Autodesk Inventor part; units mm, degrees
ref_plane "YZ Plane" through (0, 0, 0) normal (1, 0, 0) x (0, 1, 0)
ref_plane "XZ Plane" through (0, 0, 0) normal (0, 1, 0) x (-1, 0, 0)
ref_plane "XY Plane" through (0, 0, 0) normal (0, 0, 1) x (1, 0, 0)
sketch "Sketch1" plane through (0, 0, 0) normal (0, 0, 1) x (1, 0, 0)
  circle A0 centre (0, 0) radius 12
  circle A1 centre (0, 0) radius 9 construction
  circle A2 centre (9, 0) radius 1.5
  circle A3 centre (-4.5, -7.7942) radius 1.5
  circle A4 centre (-4.5, 7.7942) radius 1.5
  line L0 (9, 0) -> (-4.5, -7.7942) construction
  line L1 (-4.5, 7.7942) -> (-4.5, -7.7942) construction
  line L2 (9, 0) -> (-4.5, 7.7942) construction
  circle A5 centre (0, 0) radius 2.5
  dimension "d0" = 24
  dimension "d1" = 18
  dimension "d2" = 3
  dimension "d3" = 5
extrude "Extrusion1" add sketch "Sketch1" along normal blind 5
sketch "Sketch2" plane through (0, 0, 5) normal (0, 0, 1) x (1, 0, 0)
  circle A0 centre (9, 0) radius 2.5
  circle A1 centre (-4.5, 7.7942) radius 2.5
  circle A2 centre (-4.5, -7.7942) radius 2.5
  circle A3 centre (9, 0) radius 1.5
  circle A4 centre (-4.5, -7.7942) radius 1.5
  circle A5 centre (-4.5, 7.7942) radius 1.5
  circle A6 centre (0, 0) radius 4
  circle A7 centre (0, 0) radius 2.5
  circle A8 centre (0, 0) radius 6.5
  dimension "d6" = 5
  dimension "d7" = 8
  dimension "d12" = 13
extrude "Extrusion2" cut sketch "Sketch2" against normal blind 3 contours A0 | A2 | A1 | A5
extrude "Extrusion3" add sketch "Sketch2" along normal blind 9 contours A6
sketch "Sketch3" plane through (0, 0, 0) normal (0, 0, -1) x (-1, 0, 0)
  circle A0 centre (0, 0) radius 12
  circle A1 centre (0, 0) radius 5.5
  dimension "d13" = 11
extrude "Extrusion4" cut sketch "Sketch3" against normal blind 3 contours A1
sketch "Sketch4" plane through (0, 0, 14) normal (0, 0, 1) x (1, 0, 0)
  circle A0 centre (0, 0) radius 4
  circle A1 centre (0, 0) radius 2.5
  line L0 (-0.2, -4) -> (-0.2, 4)
  line L1 (-0.2, 4) -> (0.2, 4)
  line L2 (0.2, 4) -> (0.2, -4)
  line L3 (0.2, -4) -> (-0.2, -4)
  point P0 (0, -4)
  point P1 (0, 4)
  point P2 (0.2, -2.492)
  point P3 (0.2, -3.995)
  point P4 (0.2, 3.995)
  point P5 (0.2, 2.492)
  point P6 (-0.2, 2.492)
  point P7 (-0.2, 3.995)
  point P8 (-0.2, -3.995)
  point P9 (-0.2, -2.492)
  dimension "d16" = 0.4
extrude "Extrusion5" add sketch "Sketch4" along normal blind 13 contours A0 L2 A1 | L0 A1 A0
properties part number "Bearing_Mount"
Part model, mm, in its own coordinate system. A direction names the side the tool comes from. Give positions to 0.01 mm unless a question says otherwise; leave off trailing zeros. Order: outer loops, then holes, each group sorted by start corner. A loop starts at its lowest first (then second) coordinate and runs counter-clockwise, first axis right, second up. Notation, with made-up numbers: M 67,80.25 L 104,80.25 A31 ccw 104,110.25 Z; hole C 69.25,31.5 d4. An arc over 180 degrees is marked long. Use a Markdown table: item, result. Add a question column.
(1) Mould opens along Y. For faces 4 (the face through (-3, 3, 5)), 5 (the face through (-11.99, -0.53, 2.46)), 6 (the face through (-3.3, 5.6, 3.5)) say: +Y half, -Y half, draft (parallel to the pull), parting line (faces both ways), or undercut.
(2) Probe line 1 along Y through (x, z) = (-4.5, 0.95); line 2 along Y through (x, z) = (0, 13); line 3 along X through (y, z) = (-0.25, 25). List the from-to ranges inside material, lowest first. Write a range as [from, to].
(3) Drop flat-ended pins along their axis: P1, Ø10, axis at x = -8.5, z = 21.5, coming from the +Y side; P2, Ø10, axis at x = 6.5, z = 7.5, coming from the -Y side; P3, Ø4, axis at x = 9, y = 0, coming from the +Z side. Give the stop position or say it passes through.
(4) Saw through at D-D, the plane y = -9.75. Give the cut face in (x, z), and give its area (3 significant figures).
(5) 3-axis set-ups, long thin cutter, end or side, ignore diameter. For faces 1 (the face through (0.2, 3, 20)), 2 (the face through (9, -2, 2)), 3 (the face through (3, 0, 3)): which of +Z, -Z, +X, -X, +Y, -Y reach the whole face in a straight line?
(6) Saw through at C-C, the plane y = -1. Give the cut face in (x, z), and give its area (3 significant figures).
(7) Saw through at B-B, the plane x = -4.5. Give the cut face in (y, z).
(8) Saw through at A-A, the plane z = 18.75. Give the cut face in (x, y) (3 decimals).
Answer key:
| question | item | result |
|---|---|---|
| 1 | face 4 | draft |
| 1 | face 5 | parting line |
| 1 | face 6 | undercut |
| 2 | line 1 | [-11.12, -9.29], [-6.29, -3.16], [3.16, 6.29], [9.29, 11.12] |
| 2 | line 2 | [-4, -2.5], [2.5, 4] |
| 2 | line 3 | [-3.99, -2.49], [2.49, 3.99] |
| 3 | P1 | y = 1.94 |
| 3 | P2 | y = -11.8 |
| 3 | P3 | z = 2 |
| 4 | outline | M -7,0 L 7,0 L 7,5 L -2.94,5 L -2.94,2 L -6.06,2 L -6.06,5 L -7,5 Z |
| 4 | area | 60.6 mm^2 |
| 5 | face 1 | +Z, +Y, -Y |
| 5 | face 2 | +Z |
| 5 | face 3 | -Z |
| 6 | outline | M -11.96,0 L -5.41,0 L -5.41,3 L -2.29,3 L -2.29,27 L -3.87,27 L -3.87,5 L -11.96,5 Z; M 2.29,3 L 5.41,3 L 5.41,0 L 7.88,0 L 7.88,2 L 6.71,2 L 6.71,5 L 3.87,5 L 3.87,27 L 2.29,27 Z; M 10.12,0 L 11.96,0 L 11.96,5 L 11.29,5 L 11.29,2 L 10.12,2 Z |
| 6 | area | 129 mm^2 |
| 7 | outline | M -11.12,0 L -9.29,0 L -9.29,2 L -10.29,2 L -10.29,5 L -11.12,5 Z; M -6.29,0 L -3.16,0 L -3.16,3 L 3.16,3 L 3.16,0 L 6.29,0 L 6.29,2 L 5.29,2 L 5.29,5 L -5.29,5 L -5.29,2 L -6.29,2 Z; M 9.29,0 L 11.12,0 L 11.12,5 L 10.29,5 L 10.29,2 L 9.29,2 Z |
| 8 | outline | M -0.2,-3.995 L -0.2,-2.492 A2.5 cw -0.2,2.492 L -0.2,3.995 A4 ccw Z; M 0.2,-3.995 A4 ccw 0.2,3.995 L 0.2,2.492 A2.5 cw 0.2,-2.492 Z |
